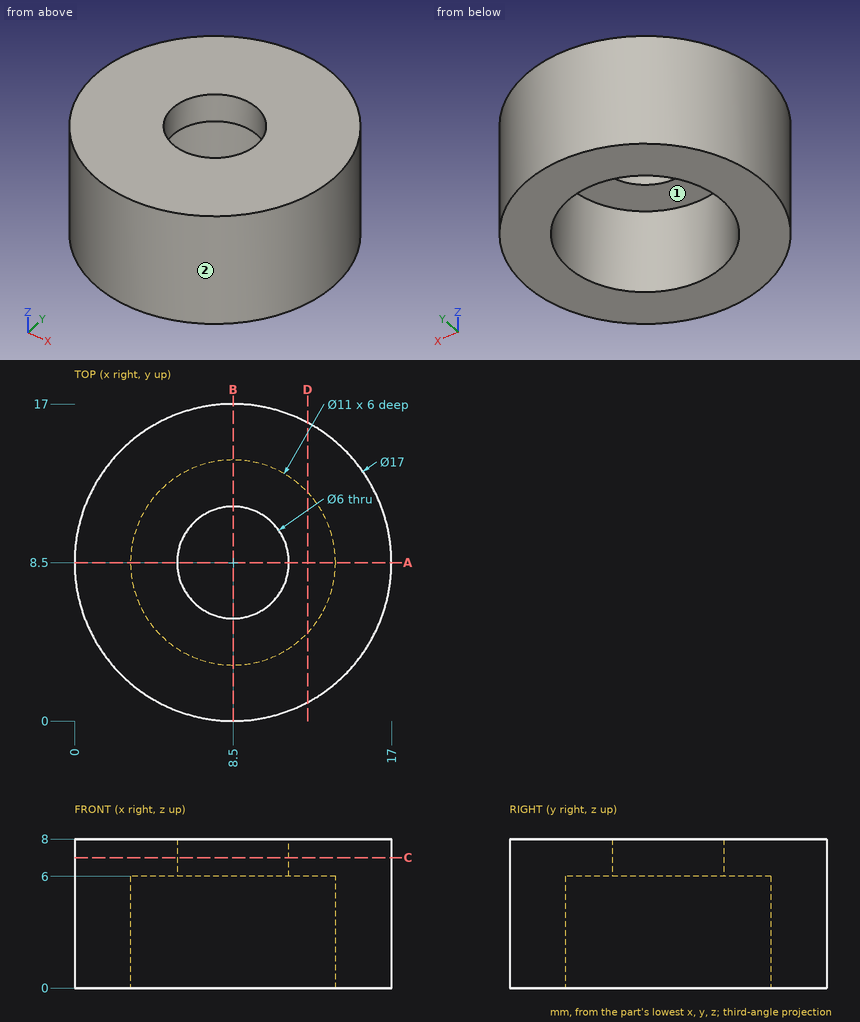
Geometry: see drawing. Coordinates: mm, zero at the bounding-box minimum. A direction names the side the tool comes from. Coordinates: 2 decimals unless noted, no trailing zeros. Write each loop counter-clockwise with the first axis right and the second up, starting at its lowest first coordinate (ties: lowest second). Pieces come first, ordered by that corner, then holes. Notation, with made-up numbers: (7, 20.25) - (38, 20.25) arc R25 ccw to (38, 34.25) - close; hole circle Ø11 at (61.25, -8.5). An arc over 180 degrees is marked (long way). Put each result on its own line as item: value. Start each with the question number.
1) Reachability of the marked faces 1 and 2 from +Z, -Z, +X, -X, +Y, -Y: full face, straight path, thin tool, end or side. Return the list, or none.
2) Contact query for flat-ended pins moving along their axis: pin 1 (1 mm diameter, centred on x = 12.5, z = 2.5, fed in from +Y); pin 2 (1 mm diameter, centred on x = 13.5, z = 1.5, fed in from -Y); pin 3 (1 mm diameter, centred on x = 9.5, z = 2, fed in from +Y). Output: stop coordinate, or through.
3) Cut plane D-D (x = 12.5). Return the cut outline in (y, z), plus the area to 3 significant figures.
4) Ray query, L1, parallel to Y at x = 8.5, z = 1.8; L2, parallel to Y at x = 8.5, z = 7.4; L3, parallel to X at y = 6.75, z = 5.5. Return the intervals inside material, ascending.
5) Cut plane A-A (y = 8.5). Return the cut outline in (x, z), plus the area to 3 significant figures.
6) Cut plane C-C (z = 7). Return the cut outline in (x, y).
Resolved:
1. face 1: -Z
1. face 2: +Z, -Z
2. pin 1: stops at y = 16.25
2. pin 2: stops at y = 1.29
2. pin 3: stops at y = 16.99
3. outline: (1, 0) - (4.73, 0) - (4.73, 6) - (12.27, 6) - (12.27, 0) - (16, 0) - (16, 8) - (1, 8) - close
3. area: 74.7 mm2
4. L1: y = 0 to 3, 14 to 17
4. L2: y = 0 to 5.5, 11.5 to 17
4. L3: x = 0.18 to 3.29, 13.71 to 16.82
5. outline: (0, 0) - (3, 0) - (3, 6) - (5.5, 6) - (5.5, 8) - (0, 8) - close; (11.5, 6) - (14, 6) - (14, 0) - (17, 0) - (17, 8) - (11.5, 8) - close
5. area: 58.0 mm2
6. outline: circle Ø17 at (8.5, 8.5); hole circle Ø6 at (8.5, 8.5)
